The model under review builds one solid part; all positions refer to its coordinate system, in mm. A direction names the side the tool comes from. Round coordinates to 2 decimals unless told otherwise and drop trailing zeros. Order: outer loops, then holes, each group sorted by start corner. A loop starts at its lowest first (then second) coordinate and runs counter-clockwise, first axis right, second up.
from build123d import *

# Parameters (mm, degrees)
SKETCH1_R           = 4.2164
BOSS_EXTRUDE1_DEPTH = 3.175


with BuildPart() as part:
    # Sketch1 → Boss-Extrude1 (new body)
    with BuildSketch(Plane(origin=(0, 0, 0), x_dir=(1, 0, 0), z_dir=(0, 1, 0))):
        with BuildLine():
            Line((-59.214911513, -6.894399988), (-37.765667105, 11.103653083))
            ThreePointArc((-37.765667105, 11.103653083), (-35.575837048, 11.794103848), (-33.539170947, 10.733882583))
            Line((-33.539170947, 10.733882583), (-24.735247395, 0.241775061))
            add(Edge.make_bspline(
                [(-24.735247395, 0.241775061), (-19.166526074, -6.39476858), (-1.252557909, -8.912412619)],
                knots=[0.363872068, 0.363872068, 0.363872068, 1.570796327, 1.570796327, 1.570796327], degree=2, weights=[1, 0.823375807, 1]))
            ThreePointArc((-1.252557909, -8.912412619), (8.599251475, -2.655724773), (3.991123209, 8.066655784))
            Line((3.991123209, 8.066655784), (-28.298515993, 24.042536234))
            ThreePointArc((-28.298515993, 24.042536234), (-31.966211418, 25.358907325), (-35.837304276, 25.805519754))
            Line((-35.837304276, 25.805519754), (-100.837304276, 25.805519754))
            ThreePointArc((-100.837304276, 25.805519754), (-105.526927742, 25.145881798), (-109.852615487, 23.218158783))
            Line((-109.852615487, 23.218158783), (-134.772811817, 7.630220662))
            ThreePointArc((-134.772811817, 7.630220662), (-137.279926323, -5.291755165), (-124.214911513, -6.894399988))
            Line((-124.214911513, -6.894399988), (-102.765667105, 11.103653083))
            ThreePointArc((-102.765667105, 11.103653083), (-100.575837048, 11.794103848), (-98.539170947, 10.733882583))
            Line((-98.539170947, 10.733882583), (-89.735247395, 0.241775061))
            add(Edge.make_bspline(
                [(-89.735247395, 0.241775061), (-84.166526074, -6.39476858), (-66.252557909, -8.912412619)],
                knots=[0.363872068, 0.363872068, 0.363872068, 1.570796327, 1.570796327, 1.570796327], degree=2, weights=[1, 0.823375807, 1]))
            ThreePointArc((-66.252557909, -8.912412619), (-62.519263798, -8.651355263), (-59.214911513, -6.894399988))
        make_face()
        with Locations(Location((0, 0, 0), (0, 0, 270))):
            Circle(SKETCH1_R, mode=Mode.SUBTRACT)
        with Locations(Location((-65, 0, 0), (0, 0, 270))):
            Circle(SKETCH1_R, mode=Mode.SUBTRACT)
        with Locations(Location((-130, 0, 0), (0, 0, 270))):
            Circle(SKETCH1_R, mode=Mode.SUBTRACT)
    extrude(amount=BOSS_EXTRUDE1_DEPTH)


solid = part.part
(1) We need section C-C (y = 1). Count the separate pieces of the cut face and the enclosed holes in it, and give its area (3 significant figures).
(2) To check wall thickness, follow L1, parallel to X at y = 2.5, z = 0; L2, parallel to X at y = 0.75, z = -11; L3, parallel to X at y = 1.65, z = 2.5. State the ranges of each line that lie inside material, in increasing order.
(3) We need section A-A (x = -65). Give the boundary of the cut face in (y, z) (3 decimals).
(4) The part is to be moulded in two halves that separate along X. For faces 3 (the flat face through (-122.14, 1.57, -15.53)), 4 (the flat face through (-66, 0, -13)), 5 (the flat face through (-29.2, 1.57, -5.56)), say which applies: pulls with the +X half, pulls with the -X half, needs draft (parallel to the pull), parting line crosses it, or undercut.
(5) We need section B-B (z = -6). Give the boundary of the cut face in (x, y) (3 decimals).
(6) Clearance check with a flat-ended pin moving along its axis: P1, Ø1.5, axis at x = -25.5, y = 0.5, coming from the -Z side. State where the tip first meets the part, or that it passes through.
(7) Tool access review of faces 1 (the flat face through (-48.64, 1.57, -1.98)), 2 (the flat face through (-66, 3.175, -13)): name each direction out of +Z, -Z, +X, -X, +Y, -Y from which nothing blocks a thin tool from reaching the whole face with its end or side.
(8) We need section D-D (x = -130). Give the boundary of the cut face in (y, z) (3 decimals).
Verdict:
1. separate pieces: 1
1. enclosed holes: 3
1. area: 3,110 mm2
2. L1: x = -139 to -134.22, -125.78 to -116, -89.52 to -69.22, -60.78 to -51, -24.52 to -4.22, 4.22 to 9
2. L2: x = -129.39 to -102.89, -98.79 to -37.89, -33.79 to -1.94
2. L3: x = -138.65 to -133.4, -126.6 to -118.98, -86.43 to -68.4, -61.6 to -53.98, -21.43 to -3.4, 3.4 to 8.65
3. outline: (0, -25.806) - (3.175, -25.806) - (3.175, -4.216) - (0, -4.216) - close; (0, 4.216) - (3.175, 4.216) - (3.175, 9) - (0, 9) - close
4. face 3: pulls with the -X half
4. face 4: needs draft
4. face 5: undercut
5. outline: (-136.708, 0) - (-108.848, 0) - (-108.848, 3.175) - (-136.708, 3.175) - close; (-94.567, 0) - (-43.848, 0) - (-43.848, 3.175) - (-94.567, 3.175) - close; (-29.567, 0) - (6.708, 0) - (6.708, 3.175) - (-29.567, 3.175) - close
6. P1: stops at z = -23.03
7. face 1: +Z, +Y, -Y
7. face 2: +Z, -Z, +X, -X, +Y
8. outline: (0, -10.616) - (3.175, -10.616) - (3.175, -4.216) - (0, -4.216) - close; (0, 4.216) - (3.175, 4.216) - (3.175, 9) - (0, 9) - close
